Work out the finished part from the listing and answer in its coordinate system (mm). Coordinates: 2 decimals unless noted, no trailing zeros. Order: outer loops, then holes, each group sorted by start corner. A loop starts at its lowest first (then second) coordinate and runs counter-clockwise, first axis right, second up.
1. Flat-ended cylindrical pins translate along their axes: pin 1 Ø3 at (x, y) = (-4.61, 5.75) entering from +Z; pin 2 Ø1.4 at (x, y) = (53.27, 13.86) entering from +Z; pin 3 Ø2 at (y, z) = (-8, 1) entering from +X. Find the tip coordinate at first contact, or state that the pin passes through.
2. The part is cut by section A-A, the plane z = 2.6. Count the separate pieces of the cut face and the enclosed holes in it, then the cut area to 3 significant figures.
3. The part is cut by section B-B, the plane y = 24. Give the vertices of the cut face in (x, z).
4. The part is cut by section C-C, the plane x = 8. Give the vertices of the cut face in (y, z), then the cut area to 3 significant figures.
5. Find the intervals of material crossed by probe 1 along Y at (x, z) = (9.5, 0.45); probe 2 along Y at (x, z) = (38, 2.5); probe 3 along Y at (x, z) = (25.5, 2.7), in increasing order.
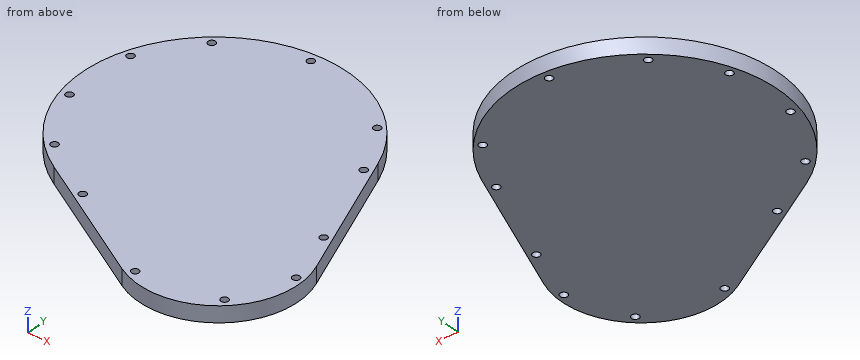
```python
from build123d import *

# Parameters (mm, degrees)
BOSS_EXTRUDE1_DEPTH        = 3.81
F_50_0_07_DIAMETER_HOLE3_D = 1.778


with BuildPart() as part:
    # Sketch1 → Boss-Extrude1 (new body)
    with BuildSketch(Plane.XY):
        with BuildLine():
            Line((0, 0), (31.187102024, -17.823710818))
            ThreePointArc((31.187102024, -17.823710818), (53.082286429, -15.709260563), (58.387158413, 5.638534012))
            Line((58.387158413, 5.638534012), (45.333427314, 39.103741383))
            ThreePointArc((45.333427314, 39.103741383), (-4.983807045, 51.60744456), (0, 0))
        make_face()
    extrude(amount=BOSS_EXTRUDE1_DEPTH)

    # #50 (0.07) Diameter Hole3 (through all)
    with Locations(Plane.XY.offset(3.81)):
        with Locations((-3.770169746, 50.098384989), (14.127303317, 57.178704003), (37.679197815, 48.033291943), (57.887608334, 0.388645245), (52.380693545, -13.624486137), (33.69651837, -16.967970116), (9.898779461, -3.544865319), (-4.606040741, 5.748053387), (-13.01391957, 20.154535826), (-12.52223075, 37.166969012), (44.661179065, 35.741071433), (53.265733422, 13.860918924)):
            Hole(F_50_0_07_DIAMETER_HOLE3_D / 2)


solid = part.part
```
Geometry says:
1. pin 1: stops at z = 3.81
1. pin 2: passes through
1. pin 3: stops at x = 58.81
2. separate pieces: 1
2. enclosed holes: 12
2. area: 4,170 mm2
3. outline: (-15.8, 0) - (51.22, 0) - (51.22, 3.81) - (-15.8, 3.81) - close
4. outline: (-4.57, 0) - (58.35, 0) - (58.35, 3.81) - (-4.57, 3.81) - close
4. area: 240 mm2
5. probe 1: y = -5.43 to -4.34, -2.75 to 58.69
5. probe 2: y = -20.15 to 47.2, 48.86 to 50.22
5. probe 3: y = -14.57 to 57.78
